```python
from build123d import *

# Parameters (mm, degrees)
F0_W        = 15.5
F0_H        = 5.5
F1_DEPTH    = 20
F2_R        = 5.5
F3_DEPTH    = 5.5
F4_W        = 34
F4_H        = 34
F4_W_2      = 15.5
F4_H_2      = 5.5
F5_DEPTH    = 100
F6_T        = 5
F6_T3_DEPTH = 15.5
F6_T5_DEPTH = 25.5
F7_R        = 5.5
F8_DEPTH    = 34


# Not quite as in the source:
# - a shell that OpenCascade refuses in one call is made with other operations: the cavity is built on its own and cut out


with BuildPart() as f1:
    # F0 (on Top) → F1 (new body)
    with BuildSketch(Plane.XY):
        Rectangle(F0_W, F0_H)
    extrude(amount=F1_DEPTH)

    # F2 (on face) → F3 (cut, through all)
    with BuildSketch(Plane.XZ.offset(2.75)):
        with Locations((0, 7.5)):
            Circle(F2_R)
    extrude(amount=-F3_DEPTH, mode=Mode.SUBTRACT)

    # F4 (on face) → F5 (join)
    with BuildSketch(Plane.XY.offset(20)):
        Rectangle(F4_W, F4_H)
        Rectangle(F4_W_2, F4_H_2, mode=Mode.SUBTRACT)
        Rectangle(F4_W_2, F4_H_2)
    extrude(amount=F5_DEPTH)

    # F6: shell of thickness 5, made by hand


with BuildPart() as f6_core1:
    # F6_t2: copy of F1
    add(f1.part)

    # the walls: a layer under each face that stays
    f6_faces = [f6_core1.faces().sort_by_distance(p)[0] for p in [
        (17, 0, 70),
        (0, -17, 70),
        (0, 17, 70),
        (-11.3333333333, -11.3333333333, 20),
        (-17, 0, 70),
        (7.75, 0, 10),
        (5.1666666667, 2.75, 16.6666666667),
        (-7.75, 0, 10),
        (-5.1666666667, -2.75, 16.6666666667),
        (0, 0, 0),
        (-5.5, 0, 7.5),
    ]]
    thicken(f6_faces, amount=-F6_T, mode=Mode.SUBTRACT)

    # F6_s4 → F6_t3 (cut)
    with BuildSketch(Plane.XZ.offset(-7.75)):
        Polygon((7.8, 19.95), (7.75, 25), (2.75, 25), (2.75, 20), align=None)
        Polygon((-7.8, 19.95), (-7.75, 25), (-2.75, 25), (-2.75, 20), align=None)
    extrude(amount=F6_T3_DEPTH, mode=Mode.SUBTRACT)

    # F6_s6 → F6_t5 (cut)
    with BuildSketch(Plane.YZ.offset(-12.75)):
        Polygon((2.8, 19.95), (2.75, 25), (-2.25, 25), (-2.25, 20), align=None)
        Polygon((-2.8, 19.95), (-2.75, 25), (2.25, 25), (2.25, 20), align=None)
    extrude(amount=F6_T5_DEPTH, mode=Mode.SUBTRACT)


with BuildPart() as f1_1:
    add(f1.part)

    # what is left inside the walls is the cavity
    f6_cavity = [f6_core1.part.solids().sort_by_distance(p)[0] for p in [
        (11.95, 0, 88.333333),
    ]]
    add(f6_cavity, mode=Mode.SUBTRACT)

    # F7 (on face) → F8 (cut, through all)
    with BuildSketch(Plane(origin=(0, 17, 0), x_dir=(-1, 0, 0), z_dir=(0, 1, 0))):
        with Locations((0, 109.5)):
            Circle(F7_R)
        with Locations((-0.0251045674, 94.500021008)):
            Circle(F7_R)
        with Locations((-0.0502091347, 79.500042016)):
            Circle(F7_R)
        with Locations((-0.0753137021, 64.500063024)):
            Circle(F7_R)
        with Locations((-0.1004182694, 49.500084032)):
            Circle(F7_R)
        with Locations((-0.1255228368, 34.50010504)):
            Circle(F7_R)
    extrude(amount=-F8_DEPTH, mode=Mode.SUBTRACT)


solid = f1_1.part
```
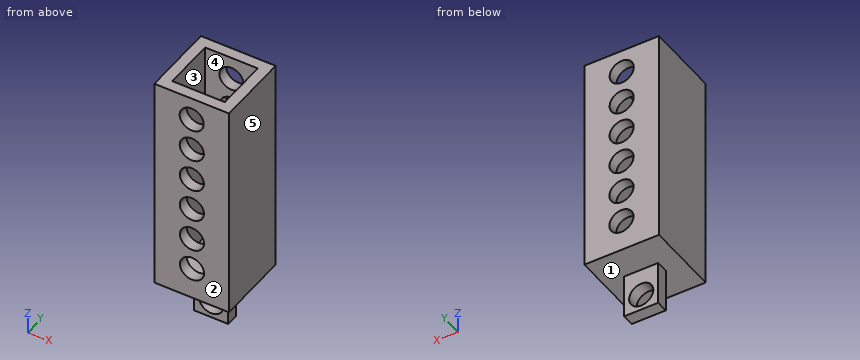
Could you check a few things on this model? Use its own coordinates, in mm. Face numbers are marked on the shaded views. A direction names the side the tool comes from. Round coordinates to 2 decimals unless told otherwise and drop trailing zeros. Write each loop counter-clockwise with the first axis right and the second up, starting at its lowest first coordinate (ties: lowest second). Pieces come first, ordered by that corner, then holes.
(1) Suppose I cut it at C-C on x = 9. Write out the boundary of the cut face in (y, z).
Findings below:
outline: (-17, 20) - (17, 20) - (17, 120) - (12, 120) - (12, 25) - (-12, 25) - (-12, 120) - (-17, 120) - close
(2) Suppose I cut it at A-A on z = 109.5. Write out the boundary of the cut face in (x, y), and give its area (3 significant figures).
Findings below:
outline: (-17, -17) - (-5.5, -17) - (-5.5, -12) - (-12, -12) - (-12, 12) - (-5.5, 12) - (-5.5, 17) - (-17, 17) - close; (5.5, -17) - (17, -17) - (17, 17) - (5.5, 17) - (5.5, 12) - (12, 12) - (12, -12) - (5.5, -12) - close
area: 470 mm2
(3) For pin 1 (17 mm diameter, centred on x = -3.5, y = 4, fed in from -Z); pin 2 (9 mm diameter, centred on x = 0, z = 109.5, fed in from -Y); pin 3 (4.5 mm diameter, centred on y = -0.5, z = 9, fed in from -X); pin 4 (1.5 mm diameter, centred on x = 8, y = 4.5, fed in from -Z), each with a flat end and sliding along its axis, tell me the tip position at first contact or that it passes through.
Findings below:
pin 1: stops at z = 0
pin 2: passes through
pin 3: stops at x = -7.75
pin 4: stops at z = 20
(4) Which directions (+Z, -Z, +X, -X, +Y, -Y) give clear straight access to the entire face, cutting with the end or side of a thin tool? Please do the marked faces 4 and 5.
Findings below:
face 4: +Z
face 5: +Z, -Z, +X, +Y, -Y
(5) If I drill on probe 1 along X at (y, z) = (0.5, 99.5); probe 2 along Z at (x, y) = (0, -0.5), over which ranges is the centre line in solid material (lowest first)?
Findings below:
probe 1: x = -17 to -12, 12 to 17
probe 2: z = 0 to 2, 13 to 25
(6) Thinking about a two-plate mould opening in Y: for the marked faces 1, 2 and 3, which applies, +Y half, -Y half, draft (parallel to the pull), parting line (faces both ways), or undercut?
Findings below:
face 1: draft
face 2: -Y half
face 3: undercut
(7) Suppose I cut it at B-B on y = 0. Write out the boundary of the cut face in (x, z), and give its area (3 significant figures).
Findings below:
outline: (-17, 20) - (-7.75, 20) - (-7.75, 0) - (7.75, 0) - (7.75, 20) - (17, 20) - (17, 120) - (12, 120) - (12, 25) - (-12, 25) - (-12, 120) - (-17, 120) - close; hole circle Ø11 at (0, 7.5)
area: 1,330 mm2
